Design review of the part built by this model. Coordinates are the model's own, in mm. A direction names the side the tool comes from. Give positions to 0.01 mm unless a question says otherwise; leave off trailing zeros. Order: outer loops, then holes, each group sorted by start corner. A loop starts at its lowest first (then second) coordinate and runs counter-clockwise, first axis right, second up. Notation, with made-up numbers: M 86,12.5 L 115,12.5 A21 ccw 115,38.5 Z; hole C 5,-38.5 d6. An arc over 180 degrees is marked long. Answer as a JSON object with one key per item and string values.
from build123d import *

# Parameters (mm, degrees)
F0_R     = 5
F0_R_2   = 3.6
F0_R_3   = 2.2
F1_DEPTH = 17.5
F0_R_4   = 9.906
F2_DEPTH = 7.5
F3_DEPTH = 5.25
F4_R     = 2
F5_R     = 0.5
F6_R     = 7
F6_R_2   = 5
F7_DEPTH = 0.5


with BuildPart() as f1:
    # F0 (on Top) → F1 (new body)
    with BuildSketch(Plane.XY):
        Circle(F0_R)
        Circle(F0_R_2, mode=Mode.SUBTRACT)
        Circle(F0_R_2)
        Circle(F0_R_3, mode=Mode.SUBTRACT)
    extrude(amount=F1_DEPTH)

    # F0 (on Top) → F2 (join)
    with BuildSketch(Plane.XY):
        Circle(F0_R_4)
        Circle(F0_R, mode=Mode.SUBTRACT)
    extrude(amount=F2_DEPTH)

    # F0 (on Top) → F3 (cut)
    with BuildSketch(Plane.XY):
        Circle(F0_R_2)
        Circle(F0_R_3, mode=Mode.SUBTRACT)
    extrude(amount=F3_DEPTH, mode=Mode.SUBTRACT)

    # F4
    f4_edges = [f1.edges().sort_by_distance(p)[0] for p in [
        (-9.906, 0, 0),
    ]]
    fillet(f4_edges, radius=F4_R)

    # F5
    f5_edges = [f1.edges().sort_by_distance(p)[0] for p in [
        (-5, 0, 17.5),
    ]]
    fillet(f5_edges, radius=F5_R)

    # F6 (on face) → F7 (join)
    with BuildSketch(Plane.XY.offset(7.5)):
        Circle(F6_R)
        Circle(F6_R_2, mode=Mode.SUBTRACT)
    extrude(amount=F7_DEPTH)


solid = f1.part
(1) Insertion check: pin 1 (3.5 mm diameter, centred on x = -0.5, y = 0.5, fed in from -Z); pin 2 (1 mm diameter, centred on x = -5, z = 13, fed in from +Y); pin 3 (2 mm diameter, centred on x = 3, z = 11, fed in from -Y). Each pin has a flat end and moves straight along its axis. Give the tip position at first contact, or say it passes through.
Checked values:
{"pin 1": "stops at z = 5.25", "pin 2": "stops at y = 2.18", "pin 3": "stops at y = -4.58"}
(2) We need section D-D (z = 9.25). Write out the cut boundary in (x, y), plus the area to 3 significant figures.
Checked values:
{"outline": "C 0,0 d10; hole C 0,0 d4.4", "area": "63.3 mm^2"}
(3) We need section A-A (x = 0). Write out the cut boundary in (y, z).
Checked values:
{"outline": "M -9.91,2 A2 ccw -7.91,0 L -3.6,0 L -3.6,5.25 L -2.2,5.25 L -2.2,17.5 L -4.5,17.5 A0.5 ccw -5,17 L -5,8 L -7,8 L -7,7.5 L -9.91,7.5 Z; M 2.2,5.25 L 3.6,5.25 L 3.6,0 L 7.91,0 A2 ccw 9.91,2 L 9.91,7.5 L 7,7.5 L 7,8 L 5,8 L 5,17 A0.5 ccw 4.5,17.5 L 2.2,17.5 Z"}
(4) Tool access review of faces 5 (the flat face through (3.4, -1.6, 0)), 6 (the flat face through (-2, -2, 5.25)), 7 (the cylindrical face through (-1.08, -4.88, 12.44)): name each direction out of +Z, -Z, +X, -X, +Y, -Y from which nothing blocks a thin tool from reaching the whole face with its end or side.
Checked values:
{"face 5": "-Z, +X, -X, +Y, -Y", "face 6": "-Z", "face 7": "+Z"}
(5) To check wall thickness, follow L1, parallel to Y at x = 0, z = 3.9; L2, parallel to Y at x = 0, z = 5.75; L3, parallel to Z at x = 1.5, y = -5.5. State the ranges of each line that lie inside material, in increasing order. Write a range as from..to.
Checked values:
{"L1": "y = -9.91..-3.6, 3.6..9.91", "L2": "y = -9.91..-2.2, 2.2..9.91", "L3": "z = 0..8"}
(6) We need section C-C (z = 6.75). Write out the cut boundary in (x, y).
Checked values:
{"outline": "C 0,0 d19.81; hole C 0,0 d4.4"}
(7) Draft analysis for pull direction X (two halves, no side actions). For faces 1 (the cylindrical face through (2.1, 0.66, 11.29)), 2 (the flat face through (-2, 5, 8)), 3 (the cylindrical face through (-1.29, 9.82, 4.71)), 4 (the cylindrical face through (3.434, 1.081, 2.588)), state which applies: +X half, -X half, draft (parallel to the pull), parting line (faces both ways), or undercut.
Checked values:
{"face 1": "undercut", "face 2": "draft", "face 3": "parting line", "face 4": "undercut"}
